Can you work these out from the model? Positions are in its coordinate system, mm. A direction names the side the tool comes from. Give positions to 0.01 mm unless a question says otherwise; leave off trailing zeros. Loops run counter-clockwise (first coordinate to the right, second up) from the corner with the lowest first, then second, coordinate; pieces in that order, holes last. Notation, with made-up numbers: M 82.5,22 L 127.5,22 A19 ccw 127.5,28 Z; hole C 30.5,-6.5 d7. An arc over 180 degrees is marked long. Use CSV: the item, a comma, the result in double quotes.
from build123d import *

# Parameters (mm, degrees)
BOSS_EXTRUDE1_DEPTH = 34
SKETCH5_R           = 11
BOSS_EXTRUDE3_DEPTH = 29.899298
SKETCH3_R           = 3
CUT_EXTRUDE1_DEPTH  = 30.899298428
FILLET1_R           = 3
CHAMFER1_SIZE       = 1


with BuildPart() as part:
    # Sketch1 → Boss-Extrude1 (new body)
    with BuildSketch(Plane.XY):
        Polygon((0, 15), (14.899298428, 15), (14.899298428, -14.949649214), (-15, -14.949649214), (-15, 15), align=None)
        Polygon((-9.966432809, 9.966432809), (-4.741432809, 9.966432809), (-3.1, 8.307461143), (-5.5, 8.307461143), (-5.5, 6.667461143), (-2.79, 3.957461143), (2.79, 3.957461143), (5.5, 6.667461143), (5.5, 8.307461143), (3.1, 8.307461143), (4.741432809, 9.966432809), (9.966432809, 9.966432809), (9.966432809, 4.741432809), (8.307461143, 3.1), (8.307461143, 5.5), (6.667461143, 5.5), (3.957461143, 2.79), (3.957461143, -2.79), (6.667461143, -5.5), (8.307461143, -5.5), (8.307461143, -3.1), (9.966432809, -4.741432809), (9.966432809, -9.966432809), (4.741432809, -9.966432809), (3.1, -8.307461143), (5.5, -8.307461143), (5.5, -6.667461143), (2.79, -3.957461143), (-2.79, -3.957461143), (-5.5, -6.667461143), (-5.5, -8.307461143), (-3.1, -8.307461143), (-4.741432809, -9.966432809), (-9.966432809, -9.966432809), (-9.966432809, -4.741432809), (-8.307461143, -3.1), (-8.307461143, -5.5), (-6.667461143, -5.5), (-3.957461143, -2.79), (-3.957461143, 2.79), (-6.667461143, 5.5), (-8.307461143, 5.5), (-8.307461143, 3.1), (-9.966432809, 4.741432809), align=None, mode=Mode.SUBTRACT)
    extrude(amount=BOSS_EXTRUDE1_DEPTH)

    # Sketch5 → Boss-Extrude3 (add, through all)
    with BuildSketch(Plane.ZY.offset(15)):
        with BuildLine():
            Line((0, 36), (0, 15))
            Line((0, 15), (0, 12.8756905))
            Line((0, 12.8756905), (34, 12.8756905))
            Line((34, 12.8756905), (34, 36))
            ThreePointArc((34, 36), (17, 53), (0, 36))
        make_face()
        with Locations((17, 36)):
            Circle(SKETCH5_R, mode=Mode.SUBTRACT)
    extrude(amount=-BOSS_EXTRUDE3_DEPTH)

    # Sketch3 → Cut-Extrude1 (cut, through all)
    with BuildSketch(Plane.ZY.offset(15)):
        with Locations((17, 0)):
            Circle(SKETCH3_R)
    extrude(amount=-CUT_EXTRUDE1_DEPTH, mode=Mode.SUBTRACT)

    # Fillet1
    fillet1_edges = [part.edges().sort_by_distance(p)[0] for p in [
        (-0.050350786, -14.949649214, 34),
        (14.899298428, 0.025175393, 34),
        (-15, 53, 17),
        (14.899298, 53, 17),
        (14.899298428, 0.025175393, 0),
        (-0.050350786, -14.949649214, 0),
        (-15, 10.525175393, 0),
        (-15, 10.525175393, 34),
        (14.899298428, -14.949649214, 17),
        (-15, -14.949649214, 17),
    ]]
    fillet(fillet1_edges, radius=FILLET1_R)

    # Chamfer1
    chamfer1_edges = [part.edges().sort_by_distance(p)[0] for p in [
        (14.899298, 36, 6),
        (-15, 36, 6),
        (14.899298428, 0, 14),
        (-15, 0, 14),
    ]]
    chamfer(chamfer1_edges, length=CHAMFER1_SIZE)


solid = part.part
Q1. Please list where these lines run through material, in increasing order: L1, parallel to Y at x = -8, z = 17; L2, parallel to Y at x = 3.25, z = 17; L3, parallel to X at y = 0, z = 10. Write a range as from..to.
Model answer:
L1,"-14.95..-9.97, -5.5..-3, 3..5.5, 9.97..25, 47..53"
L2,"-14.95..-8.46, -8.31..-4.42, 4.42..8.31, 8.46..25, 47..53"
L3,"-15..-3.96, 3.96..14.9"
Q2. I'm going to push flat-ended pins straight in: P1, Ø9.5, axis at y = 0, z = 17, coming from the +X side; P2, Ø0.8, axis at x = 7.5, z = 25.5, coming from the +Y side; P3, Ø1.6, axis at x = 6.5, z = 12, coming from the +Y side; P4, Ø5, axis at x = -7.5, y = 42, coming from the -Z side. Where does each tip first touch, or does it pass through?
Model answer:
P1,"x = 14.9"
P2,"y = 50.95"
P3,"y = 52.47"
P4,"z = 0.36"
Q3. If we mould it in two halves opening along Y, with no side actions, what happens to faces 1 (the flat face through (-9.966, -7, 17)), 2 (the cylindrical face through (-14.1, -14.09, 17.2)), 3 (the flat face through (-3.932, 9.149, 16.762))? For each: released by +Y, released by -Y, zero draft, split by the parting line, or undercut.
Model answer:
face 1,"undercut"
face 2,"released by -Y"
face 3,"undercut"
Q4. I want a section at B-B, the plane y = 0. Please give me the cut outline in (x, z), then the cut area to 3 significant figures.
Model answer:
outline,"M -15,3 A3 ccw -12,0 L -3.96,0 L -3.96,14 L -14,14 L -15,13 Z; M -15,21 L -14,20 L -3.96,20 L -3.96,34 L -12,34 A3 ccw -15,31 Z; M 3.96,0 L 11.9,0 A3 ccw 14.9,3 L 14.9,13 L 13.9,14 L 3.96,14 Z; M 3.96,20 L 13.9,20 L 14.9,21 L 14.9,31 A3 ccw 11.9,34 L 3.96,34 Z"
area,"606 mm2"
Q5. I want a section at A-A, the plane x = 0.5. Please give me the cut outline in (y, z).
Model answer:
outline,"M -14.95,3 A3 ccw -11.95,0 L -3.96,0 L -3.96,34 L -11.95,34 A3 ccw -14.95,31 Z; M 3.96,0 L 36,0 A17 ccw 36,34 L 3.96,34 Z; hole C 36,17 d22"
Q6. I want a section at C-C, the plane z = 17. State how many separate pieces and enclosed holes the cut face has, then the cut area to 3 significant figures.
Model answer:
separate pieces,"3"
enclosed holes,"0"
area,"1,050 mm2"
Q7. For faces 4 (the cylindrical face through (-0.246, 45.275, 22.914)), 5 (the flat face through (-5.5, 7, 17)), which set-ups out of +Z, -Z, +X, -X, +Y, -Y let a thin tool reach every point of the face, with its end or its side?
Model answer:
face 4,"+X, -X"
face 5,"+Z, -Z"
